Study the drawing (mm; zero at the part's minimum x, y, z) and answer. A direction names the side the tool comes from. Give positions to 0.01 mm unless a question says otherwise; leave off trailing zeros. Order: outer loops, then holes, each group sorted by start corner. A loop starts at its lowest first (then second) coordinate and runs counter-clockwise, first axis right, second up. Notation, with made-up numbers: (0.5, 8.5) -> (12.5, 8.5) arc R32 cw to (12.5, 42.5) -> close; hole circle Ø7 at (60, 37). An arc over 180 degrees is marked (long way). Answer as CSV lines item,"result". Start each with the question number.
1. A flat-ended cylindrical pin translates along its axis: pin 1 (3 mm diameter, centred on y = 5, z = 4, fed in from -X). Find the tip coordinate at first contact, or state that the pin passes through.
2. For a pull along Y with two mould halves and no side action, classify the marked faces 3, 4, 5 and 6 as released by +Y, released by -Y, zero draft, split by the parting line, or undercut.
3. For the marked faces 1 and 2, determine the directions among +Z, -Z, +X, -X, +Y, -Y from which every point of the face is accessible in a straight line to the end or side of a thin tool.
4. A cutting plane is placed at D-D (x = 6.75). Give the vertices of the cut face in (y, z).
5. A cutting plane is placed at A-A (x = 2.85). Give the vertices of the cut face in (y, z).
6. A cutting plane is placed at B-B (z = 9.2). Give the vertices of the cut face in (x, y), then the cut area to 3 significant figures.
7. A cutting plane is placed at C-C (y = 5.7). Give the vertices of the cut face in (x, z).
8. Find the intervals of material crossed by L1, parallel to Z at x = 6.7, y = 5.7; L2, parallel to Y at x = 2.85, z = 0.95; L3, parallel to Y at x = 2, z = 3, in increasing order.
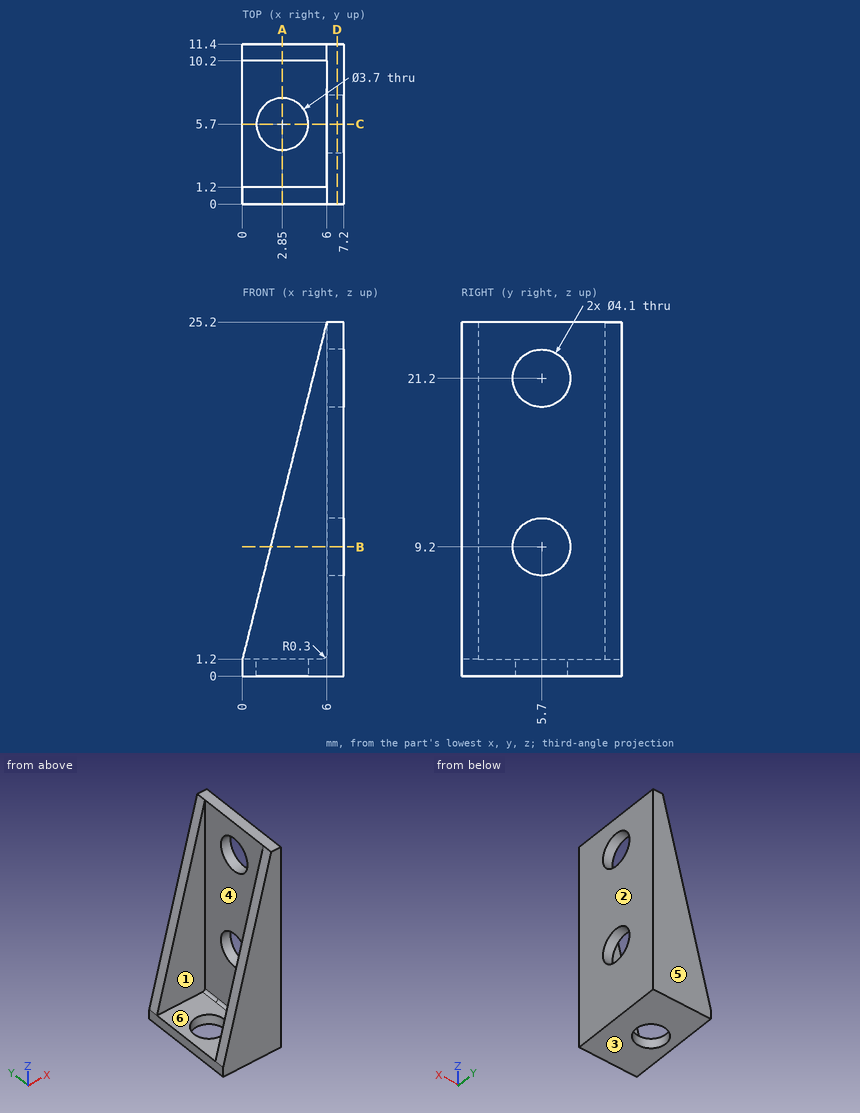
Answer sheet:
1,pin 1,"stops at x = 6"
2,face 3,"zero draft"
2,face 4,"undercut"
2,face 5,"released by +Y"
2,face 6,"undercut"
3,face 1,"+Z, -X"
3,face 2,"+Z, -Z, +X, +Y, -Y"
4,outline,"(0, 0) -> (11.4, 0) -> (11.4, 25.2) -> (0, 25.2) -> close; hole circle Ø4.1 at (5.7, 9.2); hole circle Ø4.1 at (5.7, 21.2)"
5,outline,"(0, 0) -> (3.85, 0) -> (3.85, 1.2) -> (1.2, 1.2) -> (1.2, 12.6) -> (0, 12.6) -> close; (7.55, 0) -> (11.4, 0) -> (11.4, 12.6) -> (10.2, 12.6) -> (10.2, 1.2) -> (7.55, 1.2) -> close"
6,outline,"(2, 0) -> (7.2, 0) -> (7.2, 3.65) -> (6, 3.65) -> (6, 1.2) -> (2, 1.2) -> close; (2, 10.2) -> (6, 10.2) -> (6, 7.75) -> (7.2, 7.75) -> (7.2, 11.4) -> (2, 11.4) -> close"
6,area,"18.4 mm^2"
7,outline,"(0, 0) -> (1, 0) -> (1, 1.2) -> (0, 1.2) -> close; (4.7, 0) -> (7.2, 0) -> (7.2, 7.15) -> (6, 7.15) -> (6, 1.5) arc R0.3 cw to (5.7, 1.2) -> (4.7, 1.2) -> close; (6, 11.25) -> (7.2, 11.25) -> (7.2, 19.15) -> (6, 19.15) -> close; (6, 23.25) -> (7.2, 23.25) -> (7.2, 25.2) -> (6, 25.2) -> close"
8,L1,"z = 0 to 7.15, 11.25 to 19.15, 23.25 to 25.2"
8,L2,"y = 0 to 3.85, 7.55 to 11.4"
8,L3,"y = 0 to 1.2, 10.2 to 11.4"
